```python
from build123d import *

# Parameters (mm, degrees)
SKETCH2_R           = 184.15
BOSS_EXTRUDE1_DEPTH = 6.35
SKETCH8_R           = 165.1
CUT_EXTRUDE3_DEPTH  = 261.504832009
SKETCH9_R           = 2.38125
CUT_EXTRUDE4_DEPTH  = 261.504832009
CIRPATTERN1_COUNT   = 72


with BuildPart() as part:
    # Sketch2 → Boss-Extrude1 (new body)
    with BuildSketch(Plane.XY):
        Circle(SKETCH2_R)
    extrude(amount=BOSS_EXTRUDE1_DEPTH)

    # Sketch8 → Cut-Extrude3 (cut, through all)
    with BuildSketch(Plane.XY.offset(6.35)):
        Circle(SKETCH8_R)
    extrude(amount=-CUT_EXTRUDE3_DEPTH, mode=Mode.SUBTRACT)

    # Sketch9 → Cut-Extrude4 (cut, through all)
    with BuildSketch(Plane.XY.offset(6.35)):
        with Locations((-174.049180881, 0)):
            Circle(SKETCH9_R)
    cut_extrude4 = extrude(amount=-CUT_EXTRUDE4_DEPTH, mode=Mode.SUBTRACT)

    # CirPattern1: Cut-Extrude4 ×72 about axis
    cirpattern1_axis = Axis((0, 0, 0), (0, 0, 1))
    for i in range(1, CIRPATTERN1_COUNT):
        add(cut_extrude4.rotate(cirpattern1_axis, i * 360 / CIRPATTERN1_COUNT), mode=Mode.SUBTRACT)


solid = part.part
```
Part model, mm, in its own coordinate system. Round coordinates to 2 decimals unless told otherwise and drop trailing zeros. Loops run counter-clockwise (first coordinate to the right, second up) from the corner with the lowest first, then second, coordinate; pieces in that order, holes last. Notation, with made-up numbers: (14.5, 37.25) -> (39.5, 37.25) arc R11 cw to (39.5, 44.25) -> close; hole circle Ø10 at (-22.5, 7.5). An arc over 180 degrees is marked (long way). Use a Markdown table: item, result.
1) Cut at B-B, the plane y = -22. List the corners of the cut face in (x, z), and give its area (3 significant figures).
The answers:
| item | result |
|---|---|
| outline | (-182.83, 0) -> (-163.63, 0) -> (-163.63, 6.35) -> (-182.83, 6.35) -> close; (163.63, 0) -> (182.83, 0) -> (182.83, 6.35) -> (163.63, 6.35) -> close |
| area | 244 mm2 |
2) Drop flat-ended pins along their axis: pin 1 Ø1.5 at (x, z) = (-102, 4) entering from -Y; pin 2 Ø1.5 at (y, z) = (-144, 5.5) entering from -X; pin 3 Ø2 at (y, z) = (98.5, 2) entering from -X. Give the stop position or say it passes through.
The answers:
| item | result |
|---|---|
| pin 1 | stops at y = -153.82 |
| pin 2 | stops at x = -115.72 |
| pin 3 | stops at x = -156.22 |
3) Pull direction Y, two halves, no side cores. Call faces 1 (the cylindrical face through (-146.1, -112.1, 3.1)), 2 (the cylindrical face through (-35.79, -161.174, 3.219)), 3 (the flat face through (-150.91, -67.34, 0)): pulls with the +Y half, pulls with the -Y half, needs draft (parallel to the pull), parting line crosses it, or undercut.
The answers:
| item | result |
|---|---|
| face 1 | parting line crosses it |
| face 2 | undercut |
| face 3 | needs draft |
4) Cut at A-A, the plane y = -67. List the corners of the cut face in (x, z).
The answers:
| item | result |
|---|---|
| outline | (-171.53, 0) -> (-150.89, 0) -> (-150.89, 6.35) -> (-171.53, 6.35) -> close; (150.89, 0) -> (171.53, 0) -> (171.53, 6.35) -> (150.89, 6.35) -> close |
5) Cut at C-C, the plane z = 1. State how many separate pieces and enclosed holes the cut face has, and give its area (3 significant figures).
The answers:
| item | result |
|---|---|
| separate pieces | 1 |
| enclosed holes | 73 |
| area | 19,600 mm2 |
6) Probe line 1 (X direction, y = 0.5, z = 4.75); line 2 (X direction, y = 122, z = 4.75); line 3 (Y direction, x = -89, z = 5). List the from-to ranges inside material, lowest first. Write a range as [from, to].
The answers:
| item | result |
|---|---|
| line 1 | x = [-184.15, -176.38], [-171.72, -165.1], [165.1, 171.72], [176.38, 184.15] |
| line 2 | x = [-137.94, -125.2], [-120.94, -111.24], [111.24, 120.94], [125.2, 137.94] |
| line 3 | y = [-161.21, -152.06], [-149.4, -139.06], [139.06, 149.4], [152.06, 161.21] |
